```python
from build123d import *

# Parameters (mm, degrees)
F0_W     = 25.4
F0_H     = 3.175
F1_DEPTH = 101.6
F2_R     = 2.6162
F2_R_2   = 3.302
F3_DEPTH = 3.176


with BuildPart() as f1:
    # F0 (on Front) → F1 (new body)
    with BuildSketch(Plane.XZ):
        Rectangle(F0_W, F0_H)
    extrude(amount=F1_DEPTH)

    # F2 (on face) → F3 (cut, through all)
    with BuildSketch(Plane.XY.offset(1.5875)):
        with Locations((0, -91.2876)):
            Circle(F2_R)
        with Locations((0, -10.3124)):
            Circle(F2_R)
        with Locations((0, -73.7997)):
            Circle(F2_R_2)
        with Locations((0, -27.8003)):
            Circle(F2_R_2)
    extrude(amount=-F3_DEPTH, mode=Mode.SUBTRACT)


solid = f1.part
```
The listing builds one solid part. Answer for the finished solid, in the listing's coordinates (mm). Coordinates: 2 decimals unless noted, no trailing zeros. Write each loop counter-clockwise with the first axis right and the second up, starting at its lowest first coordinate (ties: lowest second). Pieces come first, ordered by that corner, then holes. Notation, with made-up numbers: (-12, -29) - (8, -29) arc R6 cw to (8, -19) - close; hole circle Ø4 at (0.25, -29). An arc over 180 degrees is marked (long way). Return JSON: item names as keys, results as strings. Group by question number.
Q1. Find the intervals of material crossed by line 1 along Y through (x, z) = (0, -0.3); line 2 along X through (y, z) = (-72.5, 0); line 3 along X through (y, z) = (-90, 0.1), in increasing order. Write a range as [from, to].
Q2. The part is cut by section B-B on z = 0.55. Write down the section's boundary in (x, y), and give its area (3 significant figures).
Q3. For a pull along X with two mould halves and no side action, classify faces 1 (the cylindrical face through (1.52, -30.73, 0.02)), 2 (the flat face through (-12.7, -50, 0)), 3 (the flat face through (0, -50, -1.588)), 4 (the flat face through (12.7, -50, 0)) as +X half, -X half, draft (parallel to the pull), parting line (faces both ways), or undercut.
Q4. The part is cut by section A-A on x = 0. Write down the section's boundary in (y, z).
Q5. A flat-ended cylindrical pin translates along its axis: pin 1 Ø3 at (x, y) = (0, -91.29) entering from +Z. Find the tip coordinate at first contact, or state that the pin passes through.
Evaluation:
{
 "1": {"line 1": "y = [-101.6, -93.9], [-88.67, -77.1], [-70.5, -31.1], [-24.5, -12.93], [-7.7, 0]", "line 2": "x = [-12.7, -3.04], [3.04, 12.7]", "line 3": "x = [-12.7, -2.28], [2.28, 12.7]"},
 "2": {"outline": "(-12.7, -101.6) - (12.7, -101.6) - (12.7, 0) - (-12.7, 0) - close; hole circle Ø6.6 at (0, -73.8); hole circle Ø6.6 at (0, -27.8); hole circle Ø5.23 at (0, -91.29); hole circle Ø5.23 at (0, -10.31)", "area": "2,470 mm2"},
 "3": {"face 1": "undercut", "face 2": "-X half", "face 3": "draft", "face 4": "+X half"},
 "4": {"outline": "(-101.6, -1.59) - (-93.9, -1.59) - (-93.9, 1.59) - (-101.6, 1.59) - close; (-88.67, -1.59) - (-77.1, -1.59) - (-77.1, 1.59) - (-88.67, 1.59) - close; (-70.5, -1.59) - (-31.1, -1.59) - (-31.1, 1.59) - (-70.5, 1.59) - close; (-24.5, -1.59) - (-12.93, -1.59) - (-12.93, 1.59) - (-24.5, 1.59) - close; (-7.7, -1.59) - (0, -1.59) - (0, 1.59) - (-7.7, 1.59) - close"},
 "5": {"pin 1": "passes through"}
}
